Geometry: final body of the model. Coordinates: model frame, mm. A direction names the side the tool comes from. Give positions to 0.01 mm unless a question says otherwise; leave off trailing zeros. Write each loop counter-clockwise with the first axis right and the second up, starting at its lowest first coordinate (ties: lowest second). Pieces come first, ordered by that corner, then holes.
Q1. Cut plane B-B on z = 11. Return the cut outline in (x, y), plus the area to 3 significant figures.
Q2. Line query: L1, parallel to Y at x = 3.5, z = 11; L2, parallel to Y at x = 8.25, z = 11; L3, parallel to Y at x = 2, z = 17.75. Output: solid intervals per line, ascending.
Q3. Cut plane D-D on x = 5.5. Return the cut outline in (y, z).
Q4. Cut plane C-C on z = 2.75. Return the cut outline in (x, y).
Q5. Reachability of faces 1 (the face through (7, -27, 0)), 2 (the face through (7.2, -37.44, 10.85)) from +Z, -Z, +X, -X, +Y, -Y: full face, straight path, thin tool, end or side. Return the list, or none.
Q6. Draft query along Y for faces 3 (the face through (5.64, -3.07, 11.62)), 4 (the face through (0, -13, 11)), 5 (the face through (5, -59.779, 11)). Return one class per face: pulls with the +Y half, pulls with the -Y half, needs draft (parallel to the pull), parting line crosses it, or undercut.
Q7. Pin query (flat end, axial travel): pin 1 (5.5 mm diameter, centred on y = -7.78, z = 11, fed in from +X); pin 2 (2 mm diameter, centred on y = -27, z = 7.5, fed in from -X). Return the tip coordinate at first contact, or that it passes through.
Q8. Cut plane A-A on x = 8.5. Return the cut outline in (y, z), plus the area to 3 significant figures.
```python
from build123d import *

# Parameters (mm, degrees)
SKETCH_1_W          = 22
SKETCH_1_H          = 64.4
EXTRUDE_1_DEPTH     = 22
SKETCH_2_R          = 4.75
CUT_EXTRUDE_1_DEPTH = 22
SKETCH_3_W          = 22
SKETCH_3_H          = 64.4
CUT_EXTRUDE_2_DEPTH = 11


with BuildPart() as part:
    # 草圖1 → 填料-伸長1 (new body)
    with BuildSketch(Plane.XY):
        with Locations((0.13253012, -27.579314659)):
            Rectangle(SKETCH_1_W, SKETCH_1_H)
        Polygon((9.601074535, -33.279314659), (4.866802328, -25.079314659), (-4.601742087, -25.079314659), (-9.336014294, -33.279314659), (-4.601742087, -41.479314659), (4.866802328, -41.479314659), align=None, mode=Mode.SUBTRACT)
    extrude(amount=EXTRUDE_1_DEPTH)

    # 草圖2 → 除料-伸長1 (cut)
    with BuildSketch(Plane(origin=(11.13253012, 0, 0), x_dir=(0, 0, -1), z_dir=(1, 0, 0))):
        with Locations((-11, -7.779314659)):
            Circle(SKETCH_2_R)
    extrude(amount=-CUT_EXTRUDE_1_DEPTH, mode=Mode.SUBTRACT)

    # 草圖3 → 除料-伸長2 (cut)
    with BuildSketch(Plane(origin=(0, 0, 0), x_dir=(0, 0, -1), z_dir=(1, 0, 0))):
        with Locations((-11, -27.579314659)):
            Rectangle(SKETCH_3_W, SKETCH_3_H)
    extrude(amount=-CUT_EXTRUDE_2_DEPTH, mode=Mode.SUBTRACT)


solid = part.part
```
Data:
1. outline: (0, -59.78) - (11.13, -59.78) - (11.13, -12.53) - (0, -12.53) - (0, -25.08) - (4.87, -25.08) - (9.6, -33.28) - (4.87, -41.48) - (0, -41.48) - close; (0, -3.03) - (11.13, -3.03) - (11.13, 4.62) - (0, 4.62) - close
1. area: 493 mm2
2. L1: y = -59.78 to -41.48, -25.08 to -12.53, -3.03 to 4.62
2. L2: y = -59.78 to -35.62, -30.94 to -12.53, -3.03 to 4.62
2. L3: y = -59.78 to -41.48, -25.08 to 4.62
3. outline: (-59.78, 0) - (-40.38, 0) - (-40.38, 22) - (-59.78, 22) - close; (-26.18, 0) - (4.62, 0) - (4.62, 22) - (-26.18, 22) - close; hole circle Ø9.5 at (-7.78, 11)
4. outline: (0, -59.78) - (11.13, -59.78) - (11.13, 4.62) - (0, 4.62) - (0, -25.08) - (4.87, -25.08) - (9.6, -33.28) - (4.87, -41.48) - (0, -41.48) - close
5. face 1: -Z, +X, -X, +Y, -Y
5. face 2: +Z, -Z, -X
6. face 3: undercut
6. face 4: needs draft
6. face 5: pulls with the -Y half
7. pin 1: passes through
7. pin 2: stops at x = 5.4
8. outline: (-59.78, 0) - (-35.19, 0) - (-35.19, 22) - (-59.78, 22) - close; (-31.37, 0) - (4.62, 0) - (4.62, 22) - (-31.37, 22) - close; hole circle Ø9.5 at (-7.78, 11)
8. area: 1,260 mm2
